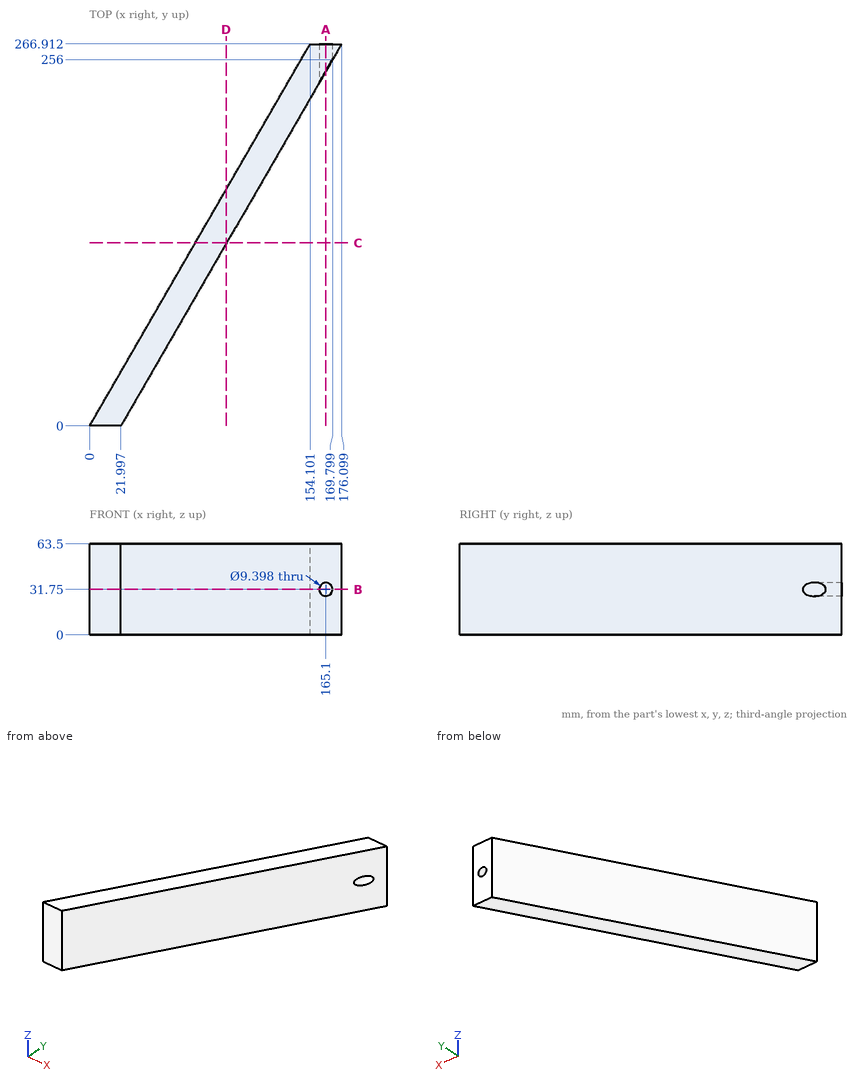
Geometry: see drawing. Coordinates: mm, zero at the bounding-box minimum. Give positions to 0.01 mm unless a question says otherwise; leave off trailing zeros. Write each loop counter-clockwise with the first axis right and the second up, starting at its lowest first coordinate (ties: lowest second). Pieces come first, ordered by that corner, then holes. Notation, with made-up numbers: (52.5, 88.5) -> (60.5, 88.5) arc R12 ccw to (60.5, 109.5) -> close; hole circle Ø8 at (69, 24.25). An arc over 180 degrees is marked (long way). Use one line per item in the form item = value. Start each with the question number.
1) Pin query (flat end, axial travel): pin 1 (2 mm diameter, centred on x = 109, z = 49.5, fed in from -Y); pin 2 (4 mm diameter, centred on y = 119.5, z = 43.5, fed in from -X); pin 3 (15 mm diameter, centred on x = 165.1, z = 31.75, fed in from -Y). Return the tip coordinate at first contact, or that it passes through.
2) Section query C-C on y = 128. Return the cut outline in (x, z), then the cut area to 3 significant figures.
3) Ray query, probe 1 along Z at (x, y) = (165.1, 251.5); probe 2 along Y at (x, z) = (39, 27.5); probe 3 along Y at (x, z) = (131.5, 25.5) (1 decimal). Return the intervals inside material, ascending. Write a range as from..to.
4) Section query A-A on x = 165.1. Return the cut outline in (y, z).
5) Section query D-D on x = 95.5. Return the cut outline in (y, z).
6) Section query B-B on z = 31.75. Return the cut outline in (x, y), then the cut area to 3 significant figures.
Outcome:
q1.pin_1 = 148.96
q1.pin_2 = 67.84
q1.pin_3 = 234.87
q2.outline = (73.9, 0) -> (95.9, 0) -> (95.9, 63.5) -> (73.9, 63.5) -> close
q2.area = 1,400 mm^2
q3.probe_1 = 0..27.05, 36.45..63.5
q3.probe_2 = 29.45..67.55
q3.probe_3 = 189.7..227.8
q4.outline = (247.86, 0) -> (266.91, 0) -> (266.91, 27.05) -> (247.86, 27.05) -> close; (247.86, 36.45) -> (266.91, 36.45) -> (266.91, 63.5) -> (247.86, 63.5) -> close
q5.outline = (127.31, 0) -> (165.41, 0) -> (165.41, 63.5) -> (127.31, 63.5) -> close
q6.outline = (0, 0) -> (22, 0) -> (160.4, 239.72) -> (160.4, 266.91) -> (154.1, 266.91) -> close; (169.8, 256) -> (176.1, 266.91) -> (169.8, 266.91) -> close
q6.area = 5,690 mm^2
